Autodesk Fusion 360 part; units mm, degrees
sketch "Mixer arm" plane through (0, 0, 0) normal (0, 0, 1) x (1, 0, 0)
  circle A0 centre (0, 0) radius 7.25
  circle A1 centre (0, 0) radius 3.25
  line L0 (-2, 65.25) -> (2, 65.25)
  line L1 (2, 65.25) -> (2, 3.25)
  line L2 (2, 3.25) -> (-2, 3.25)
  line L3 (-2, 3.25) -> (-2, 65.25)
  line L4 (-2, -3.25) -> (2, -3.25)
  line L5 (2, -3.25) -> (2, -65.25)
  line L6 (2, -65.25) -> (-2, -65.25)
  line L7 (-2, -65.25) -> (-2, -3.25)
  line L8 (-2, -7.25) -> (2, -7.25)
  line L9 (-2, 7.25) -> (2, 7.25)
  dimension "d3" = 6.5
  dimension "d5" = 14.5
  dimension "d6" = 2
  dimension "d7" = 2
  dimension "d8" = 2
  dimension "d9" = 2
  dimension "d14" = 58
  dimension "d15" = 58
extrude "Extrude1" add sketch "Mixer arm" along normal blind 3 contours A0 A1 L1 L2 L4 L5 | A0 L1 L2 L3 | A0 L1 L9 | A0 L5 L8 | A0 L4 L5 L7 | A0 L3 L9 | L0 L1 L3 L9 | A0 L7 L8 | L5 L6 L7 L8 | A0 A1 L2 L3 L4 L7
fillet "Fillet1" radius 4 4 edges at (2, -6.9687, 1.5) (2, 6.9687, 1.5) (-2, 6.9687, 1.5) (-2, -6.9687, 1.5)
fillet "Fillet2" radius 2 4 edges at (2, 65.25, 1.5) (-2, 65.25, 1.5) (-2, -65.25, 1.5) (2, -65.25, 1.5)
equation "stainless_steel_thickness = 3 mm"
equation "hole_diameter = 6.5 mm"
equation "d3 = hole_diameter"
equation "arm_thickness = 4 mm"
equation "d5 = hole_diameter + 2 * arm_thickness"
equation "d6 = arm_thickness / 2"
equation "d7 = arm_thickness / 2"
equation "d8 = arm_thickness / 2"
equation "d9 = arm_thickness / 2"
equation "d10 = stainless_steel_thickness"
equation "arm_length_front = 58 mm"
equation "arm_length_back = 58 mm"
equation "d14 = arm_length_front"
equation "d15 = arm_length_back"
equation "d17 = arm_thickness"
equation "d19 = arm_thickness / 2"
Part model, mm, in its own coordinate system. A direction names the side the tool comes from. Coordinates: 2 decimals unless noted, no trailing zeros. Write each loop counter-clockwise with the first axis right and the second up, starting at its lowest first coordinate (ties: lowest second). Pieces come first, ordered by that corner, then holes.
Item 1: Probe line 1 (Y direction, x = 0, z = 1.4); line 2 (X direction, y = -19.5, z = 1.7); line 3 (Y direction, x = -0.75, z = 0.3). List the from-to ranges inside material, lowest first.
Item 2: Which spindle directions (+Z, -Z, +X, -X, +Y, -Y) get a long thin tool onto all of the face, cutting with end or side? Do faces 1 (the face through (-2, -37, 1)), 2 (the face through (-2, 36, 1)), 3 (the face through (2, 37, 1)). Say none if no direction does.
Item 3: Slice it at C-C (x = -6). Write the cut outline in (y, z), and give its area (3 significant figures).
Item 4: Pin check, flat tips, straight feed: pin 1 (1 mm diameter, centred on y = 35, z = 0.5, fed in from -X); pin 2 (5 mm diameter, centred on x = 5.5, y = 23, fed in from -Z); pin 3 (0.9 mm diameter, centred on y = 29.5, z = 1, fed in from +X). Stop position of each tip, or through.
Item 5: Slice it at D-D (x = 5.75). Write the cut outline in (y, z).
Item 6: Mould opens along Y. For faces 4 (the face through (-2.579, 1.978, 1.479)), 5 (the face through (-1.4, 64.68, 1.52)), 6 (the face through (-3.3, 0.9, 0)) say: released by +Y, released by -Y, zero draft, split by the parting line, or undercut.
Item 7: Slice it at A-A (y = 0). Write the cut outline in (x, z).
Results found:
1. line 1: y = -65.25 to -3.25, 3.25 to 65.25
1. line 2: x = -2 to 2
1. line 3: y = -65.1 to -3.16, 3.16 to 65.1
2. face 1: +Z, -Z, -X, -Y
2. face 2: +Z, -Z, -X, +Y
2. face 3: +Z, -Z, +X, +Y
3. outline: (-4.07, 0) - (4.07, 0) - (4.07, 3) - (-4.07, 3) - close
3. area: 24.4 mm2
4. pin 1: stops at x = -2
4. pin 2: passes through
4. pin 3: stops at x = 2
5. outline: (-4.42, 0) - (4.42, 0) - (4.42, 3) - (-4.42, 3) - close
6. face 4: undercut
6. face 5: released by +Y
6. face 6: zero draft
7. outline: (-7.25, 0) - (-3.25, 0) - (-3.25, 3) - (-7.25, 3) - close; (3.25, 0) - (7.25, 0) - (7.25, 3) - (3.25, 3) - close
